The listing builds one solid part. Answer for the finished solid, in the listing's coordinates (mm). A direction names the side the tool comes from. Round coordinates to 2 decimals unless told otherwise and drop trailing zeros. Write each loop counter-clockwise with the first axis right and the second up, starting at its lowest first coordinate (ties: lowest second). Pieces come first, ordered by that corner, then holes.
Item 1: Find section B-B on x = 0. Give the vertices of the cut face in (y, z).
Item 2: For a pull along Z with two mould halves and no side action, classify faces 4 (the face through (1.32, 32.62, -29.97)), 5 (the face through (-5, 24, 3)), 6 (the face through (-12.17, 46.73, -15.87)), 7 (the face through (-52.15, 4.93, 29.99)) as +Z half, -Z half, draft (parallel to the pull), parting line (faces both ways), or undercut.
Item 3: Find section A-A on z = -25. Give the vertices of the cut face in (x, y).
Item 4: Find section D-D on x = -37. Give the vertices of the cut face in (y, z), then the cut area to 3 significant figures.
Item 5: Find section C-C on y = 26. Give the vertices of the cut face in (x, z), then the cut area to 3 significant figures.
Item 6: Each of these flat-tipped pins is pushed along its axis until it touches: pin 1 (1.5 mm diameter, centred on y = 19.5, z = 3.5, fed in from +X); pin 2 (1 mm diameter, centred on x = -11.5, y = 25.5, fed in from -Z); pin 3 (5 mm diameter, centred on y = 32, z = -11, fed in from -X). Where does it stop, or does it pass through?
Item 7: Find the intervals of material crossed by probe 1 along Z at (x, y) = (-45, 4); probe 2 along X at (y, z) = (7, 23); probe 3 along Z at (x, y) = (0, 18), in increasing order.
Item 8: A tool of negligible diameter and unlimited length cuts with its end or side. For faces 1 (the face through (0, 4, 0)), 2 (the face through (-12, 56, 22)), 3 (the face through (7, 24, -2)), from which of +Z, -Z, +X, -X, +Y, -Y can it reach the whole face along a straight path? Write none if from no direction.
```python
from build123d import *

# Parameters (mm, degrees)
SKETCH_1_R                      = 5
EXTRUDE_1_DEPTH                 = 12
CUT_EXTRUDE_START               = -2
SKETCH_3_R                      = 10
CUT_EXTRUDE_1_DEPTH             = 2
CUT_EXTRUDE_2_DEPTH             = 87.746757864
SKETCH_5_R                      = 30
SKETCH_5_R_2                    = 20
EXTRUDE_2_DEPTH                 = 54
SKETCH_6_R                      = 20
EXTRUDE_3_DEPTH                 = 16
CUT_EXTRUDE_4_DEPTH             = 8
SKETCH_7_3_R                    = 5
CUT_EXTRUDE_5_DEPTH             = 75.551995278
CUT_EXTRUDE_6_DEPTH             = 93.032602919
CUT_EXTRUDE_6_DEPTH_BACK        = 93.032602919
SKETCH_8_R                      = 12
CUT_EXTRUDE_7_REACH             = 94.033
CUT_EXTRUDE_7_END_RADIUS        = 12
CUT_EXTRUDE_7_DIRECTION_2_DEPTH = 93.032602919


with BuildPart() as part:
    # 草图1 → 凸台-拉伸1 (new body)
    with BuildSketch(Plane(origin=(0, 0, 0), x_dir=(1, 0, 0), z_dir=(0, 1, 0))):
        with BuildLine():
            Line((-45, -33), (45, -33))
            ThreePointArc((45, -33), (52.071067812, -30.071067812), (55, -23))
            Line((55, -23), (55, 23))
            ThreePointArc((55, 23), (52.071067812, 30.071067812), (45, 33))
            Line((45, 33), (-45, 33))
            ThreePointArc((-45, 33), (-52.071067812, 30.071067812), (-55, 23))
            Line((-55, 23), (-55, -23))
            ThreePointArc((-55, -23), (-52.071067812, -30.071067812), (-45, -33))
        make_face()
        with Locations(Location((-45, 23, 0), (0, 0, 270))):
            Circle(SKETCH_1_R, mode=Mode.SUBTRACT)
        with Locations(Location((45, 23, 0), (0, 0, 270))):
            Circle(SKETCH_1_R, mode=Mode.SUBTRACT)
        with Locations(Location((45, -23, 0), (0, 0, 270))):
            Circle(SKETCH_1_R, mode=Mode.SUBTRACT)
        with Locations(Location((-45, -23, 0), (0, 0, 270))):
            Circle(SKETCH_1_R, mode=Mode.SUBTRACT)
    extrude(amount=EXTRUDE_1_DEPTH)

    # 草图3 → 切除-拉伸1 (cut)
    with BuildSketch(Plane(origin=(0, 12, 0), x_dir=(1, 0, 0), z_dir=(0, 1, 0)).offset(CUT_EXTRUDE_START)):
        with Locations((-45, 23)):
            Circle(SKETCH_3_R)
        with Locations((-45, -23)):
            Circle(SKETCH_3_R)
        with Locations((45, -23)):
            Circle(SKETCH_3_R)
        with Locations((45, 23)):
            Circle(SKETCH_3_R)
    extrude(amount=CUT_EXTRUDE_1_DEPTH, mode=Mode.SUBTRACT)

    # 草图4 → 切除-拉伸2 (cut, through all)
    with BuildSketch(Plane.XY.offset(33)):
        with BuildLine():
            Line((-27.5, 0), (-27.5, 3))
            ThreePointArc((-27.5, 3), (-27.207106781, 3.707106781), (-26.5, 4))
            Line((-26.5, 4), (26.5, 4))
            ThreePointArc((26.5, 4), (27.207106781, 3.707106781), (27.5, 3))
            Line((27.5, 3), (27.5, 0))
            Line((27.5, 0), (-27.5, 0))
        make_face()
    extrude(amount=-CUT_EXTRUDE_2_DEPTH, mode=Mode.SUBTRACT)

    # 草图5 → 凸台-拉伸2 (add)
    with BuildSketch(Plane(origin=(0, 12, 0), x_dir=(1, 0, 0), z_dir=(0, 1, 0))):
        with Locations(Location((0, 0, 0), (0, 0, 270))):
            Circle(SKETCH_5_R)
        with Locations(Location((0, 0, 0), (0, 0, 270))):
            Circle(SKETCH_5_R_2, mode=Mode.SUBTRACT)
    extrude(amount=EXTRUDE_2_DEPTH)

    # 草图6 → 凸台-拉伸3 (add)
    with BuildSketch(Plane(origin=(0, 12, 0), x_dir=(1, 0, 0), z_dir=(0, 1, 0))):
        with Locations(Location((0, 0, 0), (0, 0, 270))):
            Circle(SKETCH_6_R)
    extrude(amount=EXTRUDE_3_DEPTH)

    # 草图7 → 切除-拉伸4 (cut)
    with BuildSketch(Plane(origin=(0, 28, 0), x_dir=(1, 0, 0), z_dir=(0, 1, 0))):
        with BuildLine():
            Line((5, -8), (5, 2))
            Line((5, 2), (10, 2))
            Line((10, 2), (10, 10))
            Line((10, 10), (-10, 10))
            Line((-10, 10), (-10, 2))
            Line((-10, 2), (-5, 2))
            Line((-5, 2), (-5, -8))
            ThreePointArc((-5, -8), (0, -3), (5, -8))
        make_face()
    extrude(amount=-CUT_EXTRUDE_4_DEPTH, mode=Mode.SUBTRACT)

    # 草图7<3> → 切除-拉伸5 (cut, through all)
    with BuildSketch(Plane(origin=(0, 28, 0), x_dir=(1, 0, 0), z_dir=(0, 1, 0))):
        with Locations(Location((0, -8, 0), (0, 0, 270))):
            Circle(SKETCH_7_3_R)
    extrude(amount=-CUT_EXTRUDE_5_DEPTH, mode=Mode.SUBTRACT)

    # 草图8 → 切除-拉伸6 (cut, two sides: drawn at the far end of the back side and taken through both)
    with BuildSketch(Plane.XY.offset(-CUT_EXTRUDE_6_DEPTH_BACK)):
        with Locations((0, 46)):
            Circle(SKETCH_8_R)
    extrude(amount=CUT_EXTRUDE_6_DEPTH + CUT_EXTRUDE_6_DEPTH_BACK, mode=Mode.SUBTRACT)

    # 切除-拉伸7: up to this cylinder (the profile starts outside it)
    cut_extrude_7_end = Plane(origin=(0, 46, 23.912941), z_dir=(0, 0, 1)) * Cylinder(CUT_EXTRUDE_7_END_RADIUS, 213.066, mode=Mode.PRIVATE)
    # 草图9 → 切除-拉伸7 (cut, up to the surface)
    with BuildSketch(Plane(origin=(0, 66, 0), x_dir=(1, 0, 0), z_dir=(0, 1, 0)), mode=Mode.PRIVATE) as cut_extrude_7_sk1:
        with BuildLine():
            Line((-12, -16), (-12, -27.49545417))
            ThreePointArc((-12, -27.49545417), (0, -30), (12, -27.49545417))
            Line((12, -27.49545417), (12, -16))
            ThreePointArc((12, -16), (0, -20), (-12, -16))
        make_face()
    cut_extrude_7_tool1 = extrude(cut_extrude_7_sk1.sketch, amount=-CUT_EXTRUDE_7_REACH, mode=Mode.PRIVATE) - cut_extrude_7_end
    add(cut_extrude_7_tool1.solids().sort_by_distance((0, 66, 23.912941))[0], mode=Mode.SUBTRACT)

    # 草图9 → 切除-拉伸7 direction 2 (cut)
    with BuildSketch(Plane(origin=(0, 66, 0), x_dir=(1, 0, 0), z_dir=(0, 1, 0))):
        with BuildLine():
            Line((-12, -16), (-12, -27.49545417))
            ThreePointArc((-12, -27.49545417), (0, -30), (12, -27.49545417))
            Line((12, -27.49545417), (12, -16))
            ThreePointArc((12, -16), (0, -20), (-12, -16))
        make_face()
    extrude(amount=CUT_EXTRUDE_7_DIRECTION_2_DEPTH, mode=Mode.SUBTRACT)


solid = part.part
```
Check values:
1. outline: (4, -33) - (12, -33) - (12, -30) - (34, -30) - (34, -20) - (28, -20) - (28, -10) - (20, -10) - (20, 3) - (4, 3) - close; (4, 13) - (28, 13) - (28, 20) - (34, 20) - (34, 30) - (12, 30) - (12, 33) - (4, 33) - close; (58, -30) - (66, -30) - (66, -20) - (58, -20) - close
2. face 4: parting line
2. face 5: undercut
2. face 6: undercut
2. face 7: +Z half
3. outline: (-54.8, 0) - (-49.58, 0) - (-49.58, 10) - (-54.8, 10) - close; (-40.42, 0) - (-27.5, 0) - (-27.5, 3) arc R1 cw to (-26.5, 4) - (26.5, 4) arc R1 cw to (27.5, 3) - (27.5, 0) - (40.42, 0) - (40.42, 10) - (35.2, 10) - (35.2, 12) - (16.58, 12) - (16.58, 66) - (-16.58, 66) - (-16.58, 12) - (-35.2, 12) - (-35.2, 10) - (-40.42, 10) - close; (49.58, 0) - (54.8, 0) - (54.8, 10) - (49.58, 10) - close; hole circle Ø24 at (0, 46)
4. outline: (0, -33) - (12, -33) - (12, -29) - (10, -29) - (10, -17) - (12, -17) - (12, 17) - (10, 17) - (10, 29) - (12, 29) - (12, 33) - (0, 33) - close
4. area: 744 mm2
5. outline: circle Ø60 at (0, 0); hole (-10, -10) - (10, -10) - (10, -2) - (5, -2) - (5, 8) arc R5 ccw to (-5, 8) - (-5, -2) - (-10, -2) - close
5. area: 2,530 mm2
6. pin 1: stops at x = 29.87
6. pin 2: stops at z = -27.91
6. pin 3: stops at x = -28.77
7. probe 1: z = -33 to -28, -18 to 18, 28 to 33
7. probe 2: x = -55 to -50, -40 to 40, 50 to 55
7. probe 3: z = -30 to 3, 13 to 30
8. face 1: +Z, -Z, -Y
8. face 2: +Z, +Y
8. face 3: +Y
